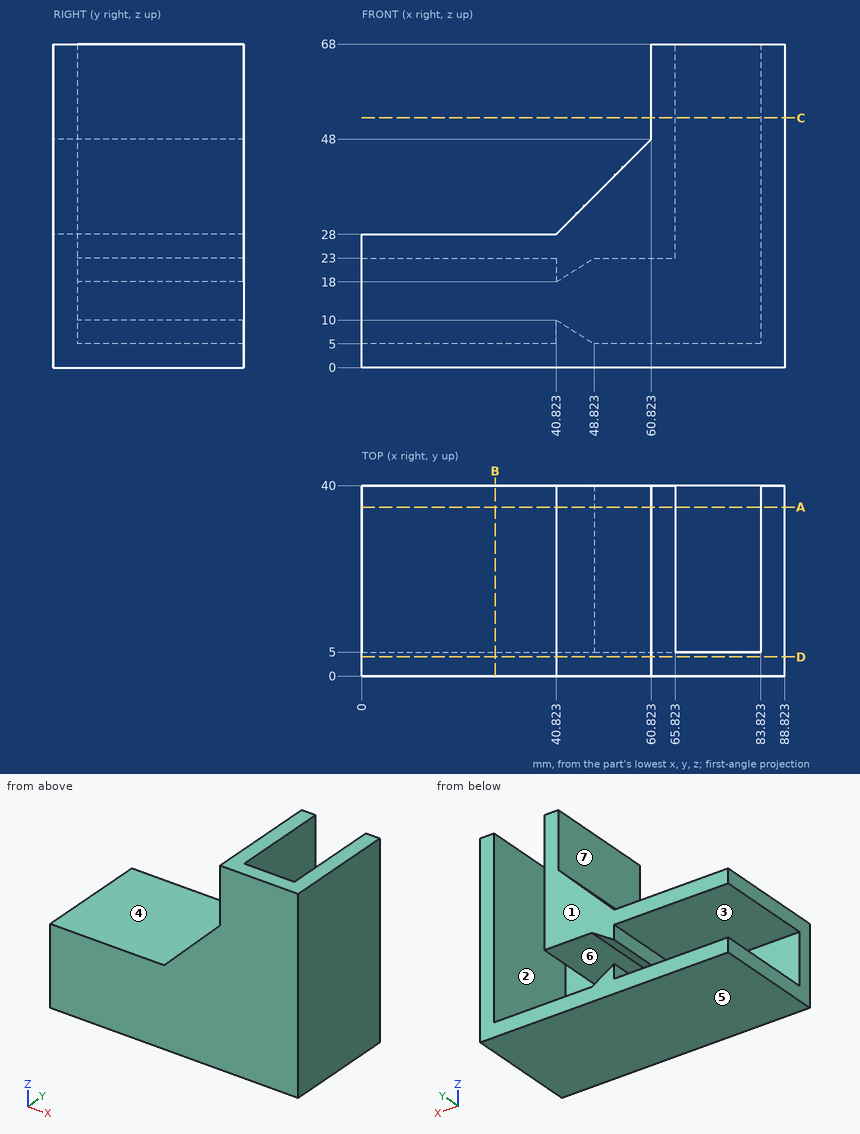
For this review, use the dimensioned drawing (mm, ordinates from the lowest corner) and the shaded views. A direction names the side the tool comes from. Coordinates: 2 decimals unless noted, no trailing zeros. Loops run counter-clockwise (first coordinate to the right, second up) from the corner with the lowest first, then second, coordinate; pieces in that order, holes last. Notation, with made-up numbers: (0.5, 64) -> (11.5, 64) arc R20 ccw to (11.5, 68) -> close; hole circle Ø6 at (1.5, 77). An arc over 180 degrees is marked (long way). Use a Markdown table: item, result. Add a question column.
1. Draft analysis for pull direction Z (two halves, no side actions). For the marked faces 4, 5, 6 and 7, state which applies: pulls with the +Z half, pulls with the -Z half, needs draft (parallel to the pull), parting line crosses it, or undercut.
2. Add section D-D on y = 4. Write out the cut boundary in (x, z).
3. Add section B-B on x = 28. Write out the cut boundary in (y, z).
4. To check wall thickness, follow line 1 (Z direction, x = 9.5, y = 22); line 2 (X direction, y = 28, z = 58); line 3 (X direction, y = 18, z = 27.5). State the ranges of each line that lie inside material, in increasing order.
5. Machinability: for the marked faces 1, 2 and 3, which of the approach directions +Z, -Z, +X, -X, +Y, -Y give a long, thin tool a straight path to every point of the face, cutting with its end or side? Answer none if there is none.
6. Add section A-A on y = 35.5. Write out the cut boundary in (x, z).
7. Clearance check with flat-ended pins moving along their axes: pin 1 Ø8 at (y, z) = (18.5, 60.5) entering from -X; pin 2 Ø1 at (y, z) = (29.5, 37) entering from -X; pin 3 Ø1.5 at (y, z) = (29.5, 7) entering from -X; pin 4 Ø10.5 at (x, y) = (71, 17) entering from +Z. State where each tip first meets the part, or that it passes through.
8. Add section C-C on z = 52.5. Write out the cut boundary in (x, y).
Returned:
| question | item | result |
|---|---|---|
| 1 | face 4 | pulls with the +Z half |
| 1 | face 5 | pulls with the -Z half |
| 1 | face 6 | undercut |
| 1 | face 7 | needs draft |
| 2 | outline | (0, 0) -> (88.82, 0) -> (88.82, 68) -> (60.82, 68) -> (60.82, 48) -> (40.82, 28) -> (0, 28) -> close |
| 3 | outline | (0, 0) -> (40, 0) -> (40, 5) -> (5, 5) -> (5, 23) -> (40, 23) -> (40, 28) -> (0, 28) -> close |
| 4 | line 1 | z = 0 to 5, 23 to 28 |
| 4 | line 2 | x = 60.82 to 65.82, 83.82 to 88.82 |
| 4 | line 3 | x = 0 to 65.82, 83.82 to 88.82 |
| 5 | face 1 | +Z, -Z, +X, -X, +Y |
| 5 | face 2 | +Z, +Y |
| 5 | face 3 | -X, +Y |
| 6 | outline | (0, 0) -> (88.82, 0) -> (88.82, 68) -> (83.82, 68) -> (83.82, 5) -> (48.82, 5) -> (40.82, 10) -> (40.82, 5) -> (0, 5) -> close; (0, 23) -> (40.82, 23) -> (40.82, 18) -> (48.82, 23) -> (65.82, 23) -> (65.82, 68) -> (60.82, 68) -> (60.82, 48) -> (40.82, 28) -> (0, 28) -> close |
| 7 | pin 1 | stops at x = 60.82 |
| 7 | pin 2 | stops at x = 49.32 |
| 7 | pin 3 | stops at x = 40.82 |
| 7 | pin 4 | stops at z = 68 |
| 8 | outline | (60.82, 0) -> (88.82, 0) -> (88.82, 40) -> (83.82, 40) -> (83.82, 5) -> (65.82, 5) -> (65.82, 40) -> (60.82, 40) -> close |
